```python
from build123d import *

# Parameters (mm, degrees)
SKETCH1_R           = 23
BOSS_EXTRUDE1_DEPTH = 5
SKETCH2_R           = 22.2
CUT_EXTRUDE1_DEPTH  = 3
SKETCH3_R           = 19.525
CUT_EXTRUDE2_DEPTH  = 7
CUT_EXTRUDE4_DEPTH  = 8
CIRPATTERN1_COUNT   = 16


with BuildPart() as part:
    # Sketch1 → Boss-Extrude1 (new body, symmetric)
    with BuildSketch(Plane.XY):
        Circle(SKETCH1_R)
    extrude(amount=BOSS_EXTRUDE1_DEPTH, both=True)

    # Sketch2 → Cut-Extrude1 (cut)
    with BuildSketch(Plane.XY.offset(5)):
        Circle(SKETCH2_R)
    extrude(amount=-CUT_EXTRUDE1_DEPTH, mode=Mode.SUBTRACT)

    # Sketch3 → Cut-Extrude2 (cut)
    with BuildSketch(Plane(origin=(0, 0, -5), x_dir=(-1, 0, 0), z_dir=(0, 0, -1))):
        Circle(SKETCH3_R)
    extrude(amount=-CUT_EXTRUDE2_DEPTH, mode=Mode.SUBTRACT)

    # Sketch5 → Cut-Extrude4 (cut)
    with BuildSketch(Plane.XY.offset(5)):
        with BuildLine():
            Line((-23, 0.75), (-21, 0.75))
            ThreePointArc((-21, 0.75), (-20.25, 0), (-21, -0.75))
            Line((-21, -0.75), (-23, -0.75))
            ThreePointArc((-23, -0.75), (-23.75, 0), (-23, 0.75))
        make_face()
    cut_extrude4 = extrude(amount=-CUT_EXTRUDE4_DEPTH, mode=Mode.SUBTRACT)

    # CirPattern1: Cut-Extrude4 ×16 about axis, 10 skipped
    cirpattern1_axis = Axis((0, 0, 5), (0, 0, 1))
    add([cut_extrude4.rotate(cirpattern1_axis, i * 360 / CIRPATTERN1_COUNT) for i in range(1, CIRPATTERN1_COUNT) if i not in (1, 2, 3, 6, 7, 8, 9, 11, 13, 14)], mode=Mode.SUBTRACT)


solid = part.part
```
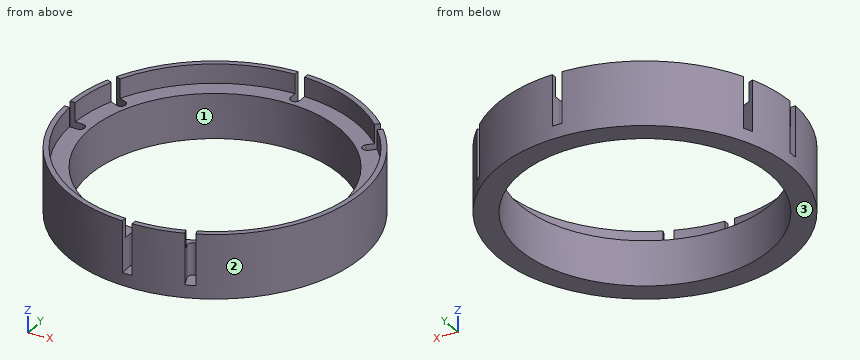
Geometry: final body of the model. Coordinates: model frame, mm. Face numbers are marked on the shaded views. Round coordinates to 2 decimals unless told otherwise and drop trailing zeros. Order: outer loops, then holes, each group sorted by start corner. A loop starts at its lowest first (then second) coordinate and runs counter-clockwise, first axis right, second up. Notation, with made-up numbers: (3.5, -19.5) -> (38.5, -19.5) arc R20 ccw to (38.5, -6.5) -> close; hole circle Ø10 at (44, 64.5). An arc over 180 degrees is marked (long way). Write each question's results on one line, items separated by ' | '.
Q1. Pull-direction query (Y, two-part tool) for the marked faces 1, 2 and 3; classes: released by +Y, released by -Y, zero draft, split by the parting line, or undercut.
Response values:
face 1: undercut | face 2: split by the parting line | face 3: zero draft
Q2. Ray query, line 1 along Y through (x, z) = (0, -2.5) (3 decimals); line 2 along X through (y, z) = (12.5, 2.75); line 3 along Y through (x, z) = (-10, 1.25). Return the intervals inside material, ascending.
Response values:
line 1: -20.25 to -19.525, 19.525 to 20.25 | line 2: -19.31 to -18.35, 18.35 to 19.31 | line 3: -20.71 to -16.77, 16.77 to 20.71
Q3. Section query C-C (y = 0). Output: boundary loops of the cut face in (x, z) (3 decimals).
Response values:
outline: (-23, -5) -> (-19.525, -5) -> (-19.525, 2) -> (-20.25, 2) -> (-20.25, -3) -> (-23, -3) -> close; (19.525, -5) -> (23, -5) -> (23, 5) -> (22.2, 5) -> (22.2, 2) -> (19.525, 2) -> close
Q4. Section query A-A (z = 3.5). Output: boundary loops of the cut face in (x, y).
Response values:
outline: (-22.99, -0.75) arc R23 ccw to (-0.75, -22.99) -> (-0.75, -22.19) arc R22.2 cw to (-22.19, -0.75) -> close; (-22.99, 0.75) -> (-22.19, 0.75) arc R22.2 cw to (-20.79, 7.8) -> (-21.52, 8.1) arc R23 ccw to start; (-20.95, 9.49) -> (-20.21, 9.18) arc R22.2 cw to (-0.75, 22.19) -> (-0.75, 22.99) arc R23 ccw to start; (0.75, -22.99) arc R23 ccw to (8.1, -21.52) -> (7.8, -20.79) arc R22.2 cw to (0.75, -22.19) -> close; (0.75, 22.19) arc R22.2 cw to (15.16, 16.22) -> (15.72, 16.79) arc R23 ccw to (0.75, 22.99) -> close; (9.18, -20.21) -> (9.49, -20.95) arc R23 ccw to (16.79, 15.72) -> (16.22, 15.16) arc R22.2 cw to start
Q5. Section query B-B (x = -3). Output: boundary loops of the cut face in (y, z).
Response values:
outline: (-22.8, -5) -> (-19.29, -5) -> (-19.29, 2) -> (-22, 2) -> (-22, 5) -> (-22.8, 5) -> close; (19.29, -5) -> (22.8, -5) -> (22.8, 5) -> (22, 5) -> (22, 2) -> (19.29, 2) -> close
Q6. Section query D-D (z = 0.25). Output: boundary loops of the cut face in (x, y) (3 decimals).
Response values:
outline: (-22.988, -0.75) arc R23 ccw to (-0.75, -22.988) -> (-0.75, -21) arc R0.75 cw to (0.75, -21) -> (0.75, -22.988) arc R23 ccw to (8.104, -21.525) -> (7.343, -19.688) arc R0.75 cw to (8.729, -19.114) -> (9.49, -20.951) arc R23 ccw to (16.785, 15.724) -> (15.38, 14.319) arc R0.75 cw to (14.319, 15.38) -> (15.724, 16.785) arc R23 ccw to (0.75, 22.988) -> (0.75, 21) arc R0.75 cw to (-0.75, 21) -> (-0.75, 22.988) arc R23 ccw to (-20.951, 9.49) -> (-19.114, 8.729) arc R0.75 cw to (-19.688, 7.343) -> (-21.525, 8.104) arc R23 ccw to (-22.988, 0.75) -> (-21, 0.75) arc R0.75 cw to (-21, -0.75) -> close; hole circle Ø39.05 at (0, 0)
Q7. Pin query (flat end, axial travel): pin 1 Ø3 at (y, z) = (-7, 0.5) entering from -X; pin 2 Ø4 at (x, z) = (-0.5, 3.5) entering from +Y; pin 3 Ø2 at (y, z) = (21.5, 3) entering from +X. Return the tip coordinate at first contact, or that it passes through.
Response values:
pin 1: x = -22.33 | pin 2: y = 22.99 | pin 3: x = 10.43
